Part model, mm, in its own coordinate system. A direction names the side the tool comes from. Coordinates: 2 decimals unless noted, no trailing zeros. Order: outer loops, then holes, each group sorted by start corner. A loop starts at its lowest first (then second) coordinate and runs counter-clockwise, first axis right, second up. Notation, with made-up numbers: M 61,35 L 75,35 A14 ccw 75,47 Z; hole C 76,73 d9. An arc over 180 degrees is marked long. Answer in a Markdown table with one row per item. Add a question column.
from build123d import *

# Parameters (mm, degrees)
SZKIC1_W                    = 64
SZKIC1_H                    = 72.64
SZKIC1_W_2                  = 52
SZKIC1_H_2                  = 18
SZKIC1_H_3                  = 2
DODANIE_WYCI_GNI_CIE1_DEPTH = 2
SFAZOWANIE1_SIZE            = 2
SZKIC2_R                    = 1.6
WYTNIJ_WYCI_GNI_CIE1_DEPTH  = 2
SZKIC3_W                    = 2.216566571
SZKIC3_H                    = 18
SZKIC3_W_2                  = 2
DODANIE_WYCI_GNI_CIE2_DEPTH = 2
WYTNIJ_WYCI_GNI_CIE2_DEPTH  = 2


with BuildPart() as part:
    # Szkic1 → Dodanie-wyciągnięcie1 (new body)
    # profile 1 of 2: a face of its own
    with BuildSketch(Plane.XY):
        with Locations((32, 36.32)):
            Rectangle(SZKIC1_W, SZKIC1_H)
        with Locations((32, 17)):
            Rectangle(SZKIC1_W_2, SZKIC1_H_2, mode=Mode.SUBTRACT)
    # profile 2 of 2: a face of its own
    with BuildSketch(Plane.XY):
        with Locations((32, 73.64)):
            Rectangle(SZKIC1_W, SZKIC1_H_3)
    extrude(amount=DODANIE_WYCI_GNI_CIE1_DEPTH)

    # Sfazowanie1
    sfazowanie1_edges = [part.edges().sort_by_distance(p)[0] for p in [
        (32, 74.64, 0),
    ]]
    chamfer(sfazowanie1_edges, length=SFAZOWANIE1_SIZE - 0.0001)  # a hair under: the kernel refuses the full size

    # Szkic2 → Wytnij-wyciągnięcie1 (cut)
    with BuildSketch(Plane.XY.offset(2)):
        with Locations((4, 30)):
            Circle(SZKIC2_R)
        with Locations((60, 30)):
            Circle(SZKIC2_R)
        with Locations((4, 68.64)):
            Circle(SZKIC2_R)
        with Locations((60, 68.64)):
            Circle(SZKIC2_R)
    extrude(amount=-WYTNIJ_WYCI_GNI_CIE1_DEPTH, mode=Mode.SUBTRACT)

    # Szkic3 → Dodanie-wyciągnięcie2 (add)
    with BuildSketch(Plane.XY.offset(2)):
        with Locations((41.891716715, 17)):
            Rectangle(SZKIC3_W, SZKIC3_H)
        with Locations((22.783433429, 17)):
            Rectangle(SZKIC3_W_2, SZKIC3_H)
    extrude(amount=-DODANIE_WYCI_GNI_CIE2_DEPTH)

    # Szkic4 → Wytnij-wyciągnięcie2 (cut)
    with BuildSketch(Plane(origin=(0, 0, 0), x_dir=(-1, 0, 0), z_dir=(0, 0, -1))):
        with BuildLine():
            Line((-48, 47.16), (-16, 47.16))
            ThreePointArc((-16, 47.16), (-11, 42.16), (-16, 37.16))
            Line((-16, 37.16), (-48, 37.16))
            ThreePointArc((-48, 37.16), (-53, 42.16), (-48, 47.16))
        make_face()
        with BuildLine():
            Line((-48, 67.48), (-16, 67.48))
            ThreePointArc((-16, 67.48), (-11, 62.48), (-16, 57.48))
            Line((-16, 57.48), (-48, 57.48))
            ThreePointArc((-48, 57.48), (-53, 62.48), (-48, 67.48))
        make_face()
    extrude(amount=-WYTNIJ_WYCI_GNI_CIE2_DEPTH, mode=Mode.SUBTRACT)


solid = part.part
(1) Pull direction X, two halves, no side cores. Call faces 3 (the flat face through (0, 37, 1)), 4 (the cylindrical face through (11, 62.6, 1)), 5 (the flat face through (32, 30, 2)): pulls with the +X half, pulls with the -X half, needs draft (parallel to the pull), parting line crosses it, or undercut.
(2) Wall check: line 1 (X direction, y = 68.64, z = 0.8); line 2 (X direction, y = 9.5, z = 1.4); line 3 (Y direction, x = 32, z = 1.6). Give the ranges that are in metal, low to high.
(3) Slice it at A-A (x = 4). State how many separate pieces and enclosed holes the cut face has, and give its area (3 significant figures).
(4) Drop a flat-ended pin along its axis: P1, Ø0.6, axis at x = 34, z = 1, coming from the +Y side. Give the stop position or say it passes through.
(5) Slice it at C-C (y = 42.16). List the corners of the cut face in (x, z), and give its area (3 significant figures).
(6) 3-axis set-ups, long thin cutter, end or side, ignore diameter. For faces 1 (the flat face through (64, 37, 1)), 2 (the flat face through (14, 26, 1)): which of +Z, -Z, +X, -X, +Y, -Y reach the whole face in a straight line?
(7) Slice it at D-D (y = 11). List the corners of the cut face in (x, z), and give its area (3 significant figures).
Computed:
| question | item | result |
|---|---|---|
| 1 | face 3 | pulls with the -X half |
| 1 | face 4 | undercut |
| 1 | face 5 | needs draft |
| 2 | line 1 | x = 0 to 2.4, 5.6 to 58.4, 61.6 to 64 |
| 2 | line 2 | x = 0 to 6, 21.78 to 23.78, 40.78 to 43, 58 to 64 |
| 2 | line 3 | y = 0 to 8, 26 to 37.16, 47.16 to 57.48, 67.48 to 74.24 |
| 3 | separate pieces | 3 |
| 3 | enclosed holes | 0 |
| 3 | area | 134 mm^2 |
| 4 | P1 | stops at y = 73.94 |
| 5 | outline | M 0,0 L 11,0 L 11,2 L 0,2 Z; M 53,0 L 64,0 L 64,2 L 53,2 Z |
| 5 | area | 44.0 mm^2 |
| 6 | face 1 | +Z, -Z, +X, +Y, -Y |
| 6 | face 2 | +Z, -Z |
| 7 | outline | M 0,0 L 6,0 L 6,2 L 0,2 Z; M 21.78,0 L 23.78,0 L 23.78,2 L 21.78,2 Z; M 40.78,0 L 43,0 L 43,2 L 40.78,2 Z; M 58,0 L 64,0 L 64,2 L 58,2 Z |
| 7 | area | 32.4 mm^2 |
